Source: CAD feature listing. Evaluate the final solid. Frame: model axes, mm. A direction names the side the tool comes from. Give positions to 0.01 mm unless a question says otherwise; leave off trailing zeros. Loops run counter-clockwise (first coordinate to the right, second up) from the corner with the lowest first, then second, coordinate; pieces in that order, holes last. Notation, with made-up numbers: M 88.25,68.25 L 135.25,68.25 A24 cw 135.25,87.25 Z; hole C 9.5,-6.5 d6. An arc over 180 degrees is marked long. Write item = value, one per line.
from build123d import *

# Parameters (mm, degrees)
SKETCH1_W           = 90
SKETCH1_H           = 110
SKETCH1_W_2         = 10
SKETCH1_H_2         = 40
SKETCH1_W_3         = 40
SKETCH1_H_3         = 10
BOSS_EXTRUDE1_DEPTH = 5
SKETCH4_R           = 20
SKETCH4_R_2         = 15.5
BOSS_EXTRUDE2_DEPTH = 10
SKETCH5_W           = 40
SKETCH5_H           = 20
BOSS_EXTRUDE3_DEPTH = 5
FILLET1_R           = 2


with BuildPart() as part:
    # Sketch1 → Boss-Extrude1 (new body)
    with BuildSketch(Plane(origin=(0, 0, 0), x_dir=(1, 0, 0), z_dir=(0, 1, 0))):
        with Locations((45, 55)):
            Rectangle(SKETCH1_W, SKETCH1_H)
        with Locations((-5, 65)):
            Rectangle(SKETCH1_W_2, SKETCH1_H_2)
        with Locations((95, 65)):
            Rectangle(SKETCH1_W_2, SKETCH1_H_2)
        with Locations((45, -5)):
            Rectangle(SKETCH1_W_3, SKETCH1_H_3)
    extrude(amount=BOSS_EXTRUDE1_DEPTH)

    # Sketch4 → Boss-Extrude2 (add)
    with BuildSketch(Plane(origin=(0, 5, 0), x_dir=(1, 0, 0), z_dir=(0, 1, 0))):
        with Locations(Location((36.72, 31.47, 0), (0, 0, 270))):
            Circle(SKETCH4_R)
        with Locations(Location((36.72, 31.47, 0), (0, 0, 270))):
            Circle(SKETCH4_R_2, mode=Mode.SUBTRACT)
    extrude(amount=BOSS_EXTRUDE2_DEPTH)

    # Sketch5 → Boss-Extrude3 (add)
    with BuildSketch(Plane(origin=(0, 5, 0), x_dir=(1, 0, 0), z_dir=(0, 1, 0))):
        with Locations((45, 110)):
            Rectangle(SKETCH5_W, SKETCH5_H)
    extrude(amount=BOSS_EXTRUDE3_DEPTH)

    # Fillet1
    fillet1_edges = [part.edges().sort_by_distance(p)[0] for p in [
        (25, 5, -105),
        (45, 5, -100),
        (65, 5, -105),
        (25, 10, -110),
        (45, 10, -100),
        (65, 10, -110),
        (45, 10, -120),
    ]]
    fillet(fillet1_edges, radius=FILLET1_R)


solid = part.part
1. Cut plane A-A, the plane z = -31.47. Return the cut outline in (x, y).
Derived:
outline = M 0,0 L 90,0 L 90,5 L 56.72,5 L 56.72,15 L 52.22,15 L 52.22,5 L 21.22,5 L 21.22,15 L 16.72,15 L 16.72,5 L 0,5 Z
2. Cut plane D-D, the plane x = 2. Return the cut outline in (y, z), then the cut area to 3 significant figures.
Derived:
outline = M 0,-110 L 5,-110 L 5,0 L 0,0 Z
area = 550 mm²
3. Reachability of faces 5 (the flat face through (77, 2, 0)), 6 (the flat face through (45, 10, -110)), 7 (the flat face through (95, 2, -85)), 8 (the flat face through (25, 7, -112)) from +Z, -Z, +X, -X, +Y, -Y: full face, straight path, thin tool, end or side. Return the list, or none.
Derived:
face_5 = +Z, +X, +Y, -Y
face_6 = -Z, +X, -X, +Y
face_7 = -Z, +X, +Y, -Y
face_8 = -Z, -X, +Y
4. Material intervals for probe 1 along X at (y, z) = (7.75, -31.47); probe 2 along Y at (x, z) = (39.5, -96.5); probe 3 along Z at (x, y) = (45, 2.5), sorted ascending. Write a range as from..to.
Derived:
probe_1 = 16.72..21.22, 52.22..56.72
probe_2 = 0..5
probe_3 = -110..10
5. First-contact query: pin 1 Ø1.5 at (y, z) = (3, 7) entering from +X; pin 2 Ø4 at (x, y) = (94.5, 3.5) entering from +Z; pin 3 Ø1.5 at (x, y) = (97, 2) entering from -Z. Flat tips, straight axial feed; report the tip coordinate or a pass-through.
Derived:
pin_1 = 65
pin_2 = -45
pin_3 = -85
6. Cut plane C-C, the plane z = -3. Return the cut outline in (x, y), then the cut area to 3 significant figures.
Derived:
outline = M 0,0 L 90,0 L 90,5 L 0,5 Z
area = 450 mm²
7. Pull-direction query (X, two-part tool) for faces 1 (the flat face through (65, 7, -112)), 2 (the flat face through (37, 5, -32)), 3 (the flat face through (0, 2, -97)), 4 (the flat face through (12, 2, 0)); classes: +X half, -X half, draft (parallel to the pull), parting line (faces both ways), or undercut.
Derived:
face_1 = +X half
face_2 = undercut
face_3 = -X half
face_4 = draft
8. Cut plane B-B, the plane x = 36.72. Return the cut outline in (y, z), then the cut area to 3 significant figures.
Derived:
outline = M 0,-110 L 5,-110 L 5,-120 L 8,-120 A2 ccw 10,-118 L 10,-102 A2 ccw 8,-100 L 7,-100 A2 cw 5,-98 L 5,-51.47 L 15,-51.47 L 15,-46.97 L 5,-46.97 L 5,-15.97 L 15,-15.97 L 15,-11.47 L 5,-11.47 L 5,10 L 0,10 Z
area = 789 mm²
